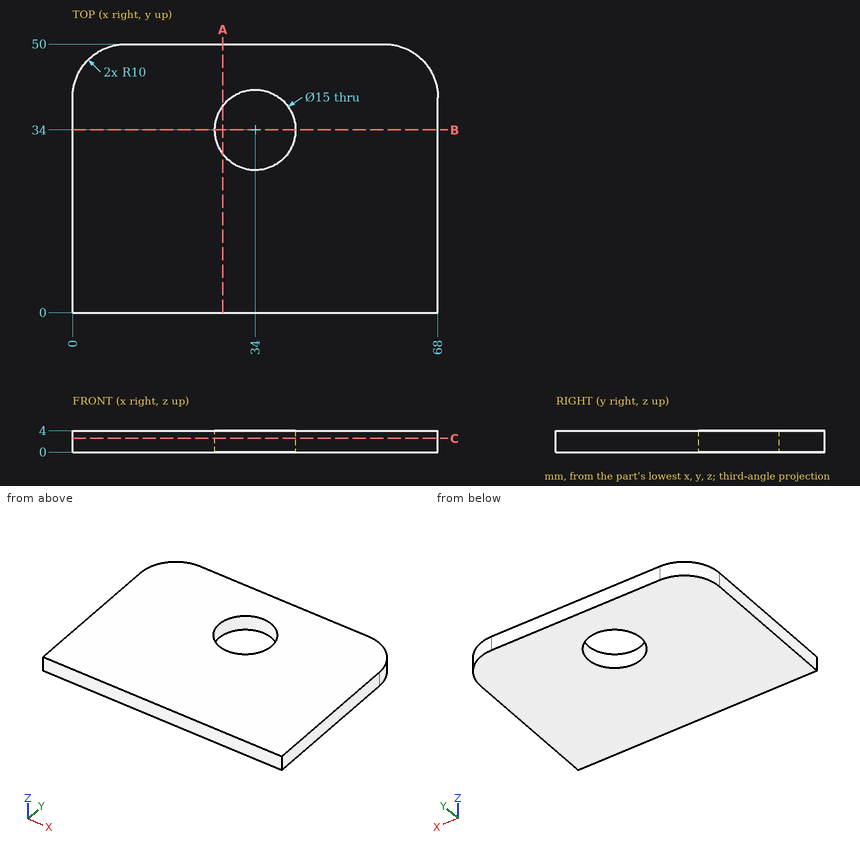
Source: three-view drawing plus pictorial views. Frame: mm from the lowest corner of the part. Coordinates: 2 decimals unless noted, no trailing zeros. Write each loop counter-clockwise with the first axis right and the second up, starting at its lowest first coordinate (ties: lowest second). Pieces come first, ordered by that corner, then holes. Notation, with made-up numbers: (65, -5) - (120, -5) arc R23 cw to (120, 16) - close; hole circle Ø8 at (-37, 7.5). An arc over 180 degrees is marked (long way). Answer as a JSON object with one key per item and string values.
Q1. Section query C-C, the plane z = 2.55. Output: boundary loops of the cut face in (x, y), plus the area to 3 significant figures.
Ans:
{"outline": "(0, 0) - (68, 0) - (68, 40) arc R10 ccw to (58, 50) - (10, 50) arc R10 ccw to (0, 40) - close; hole circle Ø15 at (34, 34)", "area": "3,180 mm2"}
Q2. Material intervals for line 1 (Y direction, x = 34, z = 3.2); line 2 (X direction, y = 38, z = 0.8); line 3 (X direction, y = 36, z = 3), sorted ascending. Write a range as [from, to].
Ans:
{"line 1": "y = [0, 26.5], [41.5, 50]", "line 2": "x = [0, 27.66], [40.34, 68]", "line 3": "x = [0, 26.77], [41.23, 68]"}
Q3. Section query A-A, the plane x = 28. Output: boundary loops of the cut face in (y, z).
Ans:
{"outline": "(0, 0) - (29.5, 0) - (29.5, 4) - (0, 4) - close; (38.5, 0) - (50, 0) - (50, 4) - (38.5, 4) - close"}
Q4. Section query B-B, the plane y = 34. Output: boundary loops of the cut face in (x, z), plus the area to 3 significant figures.
Ans:
{"outline": "(0, 0) - (26.5, 0) - (26.5, 4) - (0, 4) - close; (41.5, 0) - (68, 0) - (68, 4) - (41.5, 4) - close", "area": "212 mm2"}
